```python
from build123d import *

# Parameters (mm, degrees)
F1_DEPTH = 30
F0_W     = 4.7
F0_H     = 2.9
F2_DEPTH = 5
F3_W     = 24.7
F3_H     = 2.5
F4_DEPTH = 4


with BuildPart() as f1:
    # F0 (on Front) → F1 (new body)
    with BuildSketch(Plane.XZ):
        Polygon((-42.2, 0), (0, 0), (0, 13.7), (-17.5, 13.7), (-17.5, 8.6), (-17.5, 5.7), (-22.2, 5.7), (-22.2, 8.6), (-42.2, 8.6), align=None)
    extrude(amount=-F1_DEPTH)

    # F0 (on Front) → F2 (join)
    with BuildSketch(Plane.XZ):
        with Locations((-19.85, 7.15)):
            Rectangle(F0_W, F0_H)
    extrude(amount=-F2_DEPTH)

    # F3 (on face) → F4 (join)
    with BuildSketch(Plane.XY.offset(8.6)):
        with Locations((-29.85, 1.25)):
            Rectangle(F3_W, F3_H)
    extrude(amount=F4_DEPTH)


solid = f1.part
```
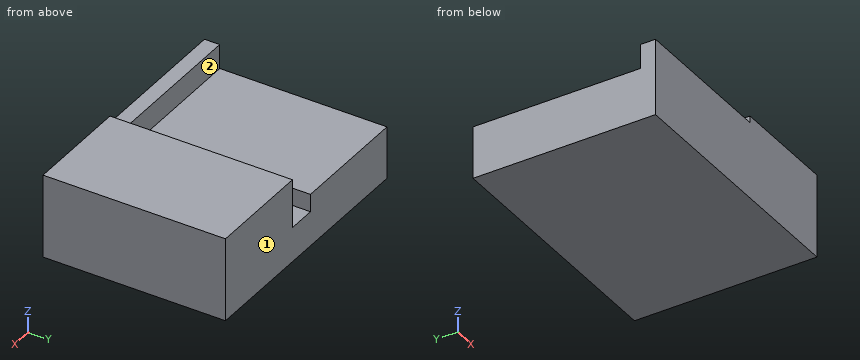
The listing builds one solid part. Answer for the finished solid, in the listing's coordinates (mm). Face numbers are marked on the shaded views. A direction names the side the tool comes from. Give positions to 0.01 mm unless a question says otherwise; leave off trailing zeros. Write each loop counter-clockwise with the first axis right and the second up, starting at its lowest first coordinate (ties: lowest second). Pieces come first, ordered by that corner, then holes. Notation, with made-up numbers: (7.5, 19) - (54.5, 19) arc R26 ccw to (54.5, 49) - close; hole circle Ø9 at (76.5, -37.5). An arc over 180 degrees is marked (long way). Use one line per item in the form item = value. Start each with the question number.
1) Consider line 1 along X through (y, z) = (16.5, 6.75); line 2 along Z through (x, y) = (-19, 19.5); line 3 along X through (y, z) = (4.5, 11.5). Determine where each line is inside the solid, lowest interval first. Write a range as from..to.
2) Find section C-C on x = -23. Determine the outline of the cut face in (y, z), plus the area to 3 significant figures.
3) Find section B-B on z = 10. Determine the outline of the cut face in (x, y).
4) Flat-ended cylindrical pins translate along their axes: pin 1 Ø3 at (x, z) = (-32, 11) entering from +Y; pin 2 Ø3 at (x, y) = (-30.5, 1.5) entering from +Z. Find the tip coordinate at first contact, or state that the pin passes through.
5) A tool of negligible diameter and unlimited length cuts with its end or side. For the marked faces 1 and 2, from which of +Z, -Z, +X, -X, +Y, -Y can it reach the whole face along a straight path? Write none if from no direction.
6) Find section A-A on y = 7.5. Determine the outline of the cut face in (x, z), plus the area to 3 significant figures.
Geometry results:
q1.line_1 = -42.2..-22.2, -17.5..0
q1.line_2 = 0..5.7
q1.line_3 = -17.5..0
q2.outline = (0, 0) - (30, 0) - (30, 8.6) - (2.5, 8.6) - (2.5, 12.6) - (0, 12.6) - close
q2.area = 268 mm2
q3.outline = (-42.2, 0) - (0, 0) - (0, 30) - (-17.5, 30) - (-17.5, 2.5) - (-42.2, 2.5) - close
q4.pin_1 = 2.5
q4.pin_2 = 12.6
q5.face_1 = +Z, -Z, +X, -X, +Y
q5.face_2 = +Z, -X, +Y
q6.outline = (-42.2, 0) - (0, 0) - (0, 13.7) - (-17.5, 13.7) - (-17.5, 5.7) - (-22.2, 5.7) - (-22.2, 8.6) - (-42.2, 8.6) - close
q6.area = 439 mm2
